from build123d import *

# Parameters (mm, degrees)
EXTRUDE_2_DEPTH     = 7
CUT_EXTRUDE_1_DEPTH = 40.702015062


with BuildPart() as part:
    # 草图1 → 凸台-拉伸2 (new body)
    with BuildSketch(Plane.XZ):
        with BuildLine():
            Line((6, 37.5), (-6, 37.5))
            ThreePointArc((-6, 37.5), (-9.535533906, 36.035533906), (-11, 32.5))
            Line((-11, 32.5), (-11, 0))
            Line((-11, 0), (11, 0))
            Line((11, 0), (11, 32.5))
            ThreePointArc((11, 32.5), (9.535533906, 36.035533906), (6, 37.5))
        make_face()
    extrude(amount=EXTRUDE_2_DEPTH)

    # 草图2 → 切除-拉伸1 (cut, through all)
    with BuildSketch(Plane(origin=(0, 0, 0), x_dir=(-1, 0, 0), z_dir=(0, 0, -1))):
        Polygon((-11, 0), (11, 0), (0, -2), align=None)
    extrude(amount=-CUT_EXTRUDE_1_DEPTH, mode=Mode.SUBTRACT)


solid = part.part
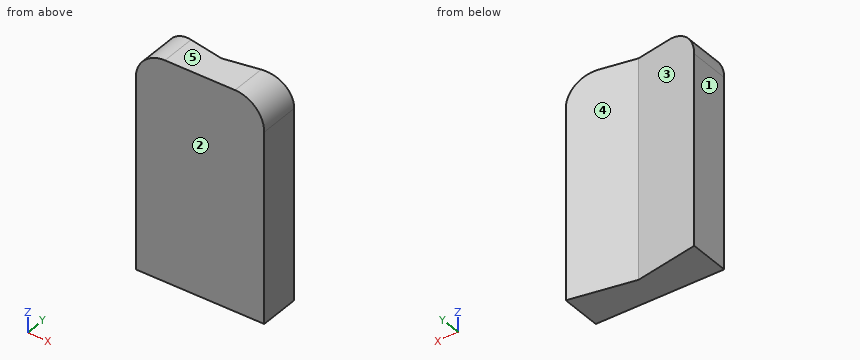
Work out the finished part from the listing and answer in its coordinate system (mm). Face numbers are marked on the shaded views. A direction names the side the tool comes from. Round coordinates to 2 decimals unless told otherwise and drop trailing zeros. Write each loop counter-clockwise with the first axis right and the second up, starting at its lowest first coordinate (ties: lowest second). Pieces come first, ordered by that corner, then holes. Notation, with made-up numbers: (27, 84.25) - (81, 84.25) arc R24 ccw to (81, 96.25) - close; hole circle Ø3 at (64.25, -4). An arc over 180 degrees is marked (long way). Answer in a Markdown table with one row per item. Add a question column.
1. Find the intervals of material crossed by line 1 along Y through (x, z) = (6, 21); line 2 along Y through (x, z) = (6.5, 21.5); line 3 along Z through (x, y) = (7, -3), in increasing order. Write a range as from..to.
2. A cutting plane is placed at A-A, the plane z = 24. Determine the outline of the cut face in (x, y), and give its area (3 significant figures).
3. The mould has two halves that part along Y. Classify the marked faces 1, 2 and 3: +Y half, -Y half, draft (parallel to the pull), parting line (faces both ways), or undercut.
4. A cutting plane is placed at C-C, the plane x = 8. Determine the outline of the cut face in (y, z).
5. A cutting plane is placed at D-D, the plane x = 2. Determine the outline of the cut face in (y, z).
6. A cutting plane is placed at B-B, the plane y = -0.5. Determine the outline of the cut face in (x, z).
7. For the marked faces 4 and 5, determine the directions among +Z, -Z, +X, -X, +Y, -Y from which every point of the face is accessible in a straight line to the end or side of a thin tool.
Worked out:
| question | item | result |
|---|---|---|
| 1 | line 1 | -7..-0.91 |
| 1 | line 2 | -7..-0.82 |
| 1 | line 3 | 0..37.4 |
| 2 | outline | (-11, -7) - (11, -7) - (11, 0) - (0, -2) - (-11, 0) - close |
| 2 | area | 132 mm^2 |
| 3 | face 1 | draft |
| 3 | face 2 | -Y half |
| 3 | face 3 | +Y half |
| 4 | outline | (-7, 0) - (-0.55, 0) - (-0.55, 37.08) - (-7, 37.08) - close |
| 5 | outline | (-7, 0) - (-1.64, 0) - (-1.64, 37.5) - (-7, 37.5) - close |
| 6 | outline | (-11, 0) - (-8.25, 0) - (-8.25, 36.97) arc R5 ccw to (-11, 32.5) - close; (8.25, 0) - (11, 0) - (11, 32.5) arc R5 ccw to (8.25, 36.97) - close |
| 7 | face 4 | +Z, -Z, +Y |
| 7 | face 5 | +Z, +X, -X, +Y, -Y |
